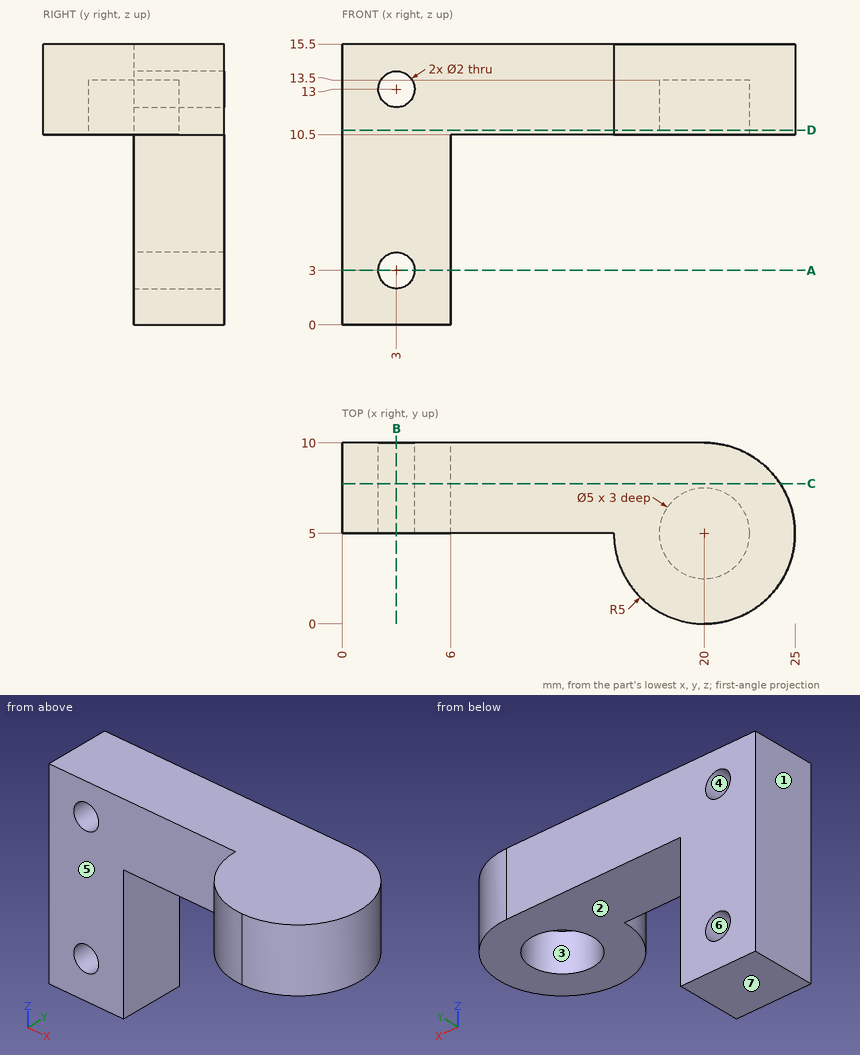
Geometry check sheet. Reference: drawing and pictorial views, mm from the part's lowest x, y, z. A direction names the side the tool comes from. Round coordinates to 2 decimals unless told otherwise and drop trailing zeros. Write each loop counter-clockwise with the first axis right and the second up, starting at its lowest first coordinate (ties: lowest second). Pieces come first, ordered by that corner, then holes.
Item 1: Mould release check, pull along Z, two halves, no side actions. Record for the marked faces 4, 5, 6 and 7: +Z half, -Z half, draft (parallel to the pull), parting line (faces both ways), or undercut.
Determined:
face 4: undercut
face 5: draft
face 6: undercut
face 7: -Z half
Item 2: Access from +Z, -Z, +X, -X, +Y, -Y to the whole of each face (thin tool, end or side, straight path). Record for the marked faces 1, 2 and 3.
Determined:
face 1: +Z, -Z, -X, +Y, -Y
face 2: -Z, +X, +Y, -Y
face 3: -Z
Item 3: Section check D-D (z = 10.75). Record the boundary of the cut face in (x, y), plus the area to 3 significant figures.
Determined:
outline: (0, 5) - (15, 5) arc R5 ccw (long way) to (20, 10) - (0, 10) - close; hole circle Ø5 at (20, 5)
area: 139 mm2
Item 4: Section check A-A (z = 3). Record the boundary of the cut face in (x, y).
Determined:
outline: (0, 5) - (2, 5) - (2, 10) - (0, 10) - close; (4, 5) - (6, 5) - (6, 10) - (4, 10) - close
Item 5: Section check C-C (y = 7.75). Record the boundary of the cut face in (x, z), plus the area to 3 significant figures.
Determined:
outline: (0, 0) - (6, 0) - (6, 10.5) - (24.18, 10.5) - (24.18, 15.5) - (0, 15.5) - close; hole circle Ø2 at (3, 3); hole circle Ø2 at (3, 13)
area: 178 mm2
Item 6: Go/stop test with flat-tipped pins: pin 1 Ø1.2 at (x, z) = (3, 3) entering from +Y; pin 2 Ø4 at (y, z) = (6.5, 4) entering from +X; pin 3 Ø3 at (x, y) = (18.5, 5) entering from -Z; pin 4 Ø7.5 at (x, z) = (9.5, 11) entering from -Y. Record where each tip stops, or that it passes through.
Determined:
pin 1: passes through
pin 2: stops at x = 6
pin 3: stops at z = 10.5
pin 4: stops at y = 5
Item 7: Section check B-B (x = 3). Record the boundary of the cut face in (y, z).
Determined:
outline: (5, 0) - (10, 0) - (10, 2) - (5, 2) - close; (5, 4) - (10, 4) - (10, 12) - (5, 12) - close; (5, 14) - (10, 14) - (10, 15.5) - (5, 15.5) - close
Item 8: Material ranges on line 1 along Z through (x, y) = (3, 8.4); line 2 along Y through (x, z) = (20, 12.2); line 3 along X through (y, z) = (7.75, 3), recorded low to high.
Determined:
line 1: z = 0 to 2, 4 to 12, 14 to 15.5
line 2: y = 0 to 2.5, 7.5 to 10
line 3: x = 0 to 2, 4 to 6
